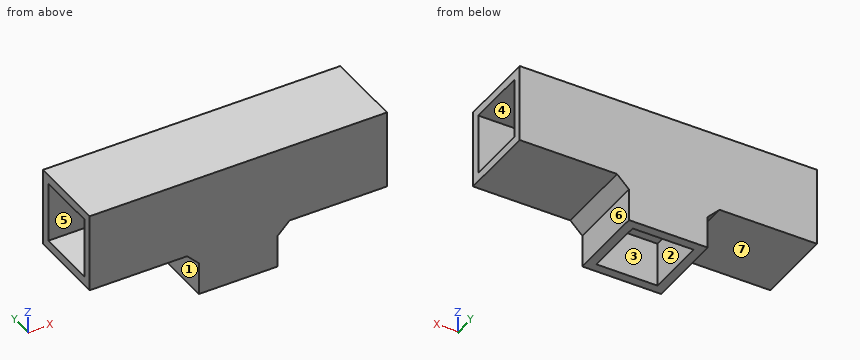
```python
from build123d import *

# Parameters (mm, degrees)
SKETCH_W      = 26.5
SKETCH_H      = 26.5
SKETCH_W_2    = 20.5
SKETCH_H_2    = 20.5
PAD_DEPTH     = 15
SKETCH001_W   = 26.5
SKETCH001_H   = 26.5
SKETCH001_W_2 = 20.5
SKETCH001_H_2 = 20.5
PAD001_DEPTH  = 50
CHAMFER_SIZE  = 4


with BuildPart() as part:
    # Sketch → Pad (new body)
    with BuildSketch(Plane.XY):
        Rectangle(SKETCH_W, SKETCH_H)
        Rectangle(SKETCH_W_2, SKETCH_H_2, mode=Mode.SUBTRACT)
    extrude(amount=PAD_DEPTH)

    # Sketch001 → Pad001 (join, symmetric)
    with BuildSketch(Plane.YZ):
        with Locations((0, 28.25)):
            Rectangle(SKETCH001_W, SKETCH001_H)
        with Locations((0, 28.25)):
            Rectangle(SKETCH001_W_2, SKETCH001_H_2, mode=Mode.SUBTRACT)
    extrude(amount=PAD001_DEPTH, both=True)

    # Chamfer
    chamfer_edges = [part.edges().sort_by_distance(p)[0] for p in [
        (13.25, 0, 15),
        (-13.25, 0, 15),
    ]]
    chamfer(chamfer_edges, length=CHAMFER_SIZE)


solid = part.part
```
The model under review builds one solid part; all positions refer to its coordinate system, in mm. Face numbers are marked on the shaded views. A direction names the side the tool comes from. Give positions to 0.01 mm unless a question says otherwise; leave off trailing zeros. Write each loop counter-clockwise with the first axis right and the second up, starting at its lowest first coordinate (ties: lowest second). Pieces come first, ordered by that corner, then holes. Notation, with made-up numbers: (-35, 43) -> (3, 43) arc R16 ccw to (3, 63) -> close; hole circle Ø7 at (43.25, -12). An arc over 180 degrees is marked (long way). Put each result on its own line as item: value.
(1) We need section D-D, the plane x = -42. Give the boundary of the cut face in (y, z), and give its area (3 significant figures).
Results are:
outline: (-13.25, 15) -> (13.25, 15) -> (13.25, 41.5) -> (-13.25, 41.5) -> close; hole (-10.25, 18) -> (10.25, 18) -> (10.25, 38.5) -> (-10.25, 38.5) -> close
area: 282 mm²
(2) For pin 1 Ø10 at (x, y) = (-1.5, -0.5) entering from -Z; pin 2 Ø9 at (y, z) = (1, 4) entering from -X; pin 3 Ø5.5 at (y, z) = (0.5, 4) entering from +X, all flat-tipped, find the tip position at first contact; note any pin that passes through.
Results are:
pin 1: z = 15
pin 2: x = -13.25
pin 3: x = 13.25
(3) We need section C-C, the plane z = 20.5. Give the boundary of the cut face in (x, y), and give its area (3 significant figures).
Results are:
outline: (-50, -13.25) -> (50, -13.25) -> (50, -10.25) -> (-50, -10.25) -> close; (-50, 10.25) -> (50, 10.25) -> (50, 13.25) -> (-50, 13.25) -> close
area: 600 mm²
(4) The part is to be moulded in two halves that separate along X. For the marked faces 1, 2, 3 and 4, say which applies: pulls with the +X half, pulls with the -X half, needs draft (parallel to the pull), parting line crosses it, or undercut.
Results are:
face 1: pulls with the -X half
face 2: undercut
face 3: undercut
face 4: needs draft
(5) Tool access review of the marked faces 5, 6 and 7: name each direction out of +Z, -Z, +X, -X, +Y, -Y from which nothing blocks a thin tool from reaching the whole face with its end or side.
Results are:
face 5: +X, -X
face 6: -Z, +X, +Y, -Y
face 7: -Z, -X, +Y, -Y
(6) We need section B-B, the plane z = 7. Give the boundary of the cut face in (x, y).
Results are:
outline: (-13.25, -13.25) -> (13.25, -13.25) -> (13.25, 13.25) -> (-13.25, 13.25) -> close; hole (-10.25, -10.25) -> (10.25, -10.25) -> (10.25, 10.25) -> (-10.25, 10.25) -> close
(7) To check wall thickness, follow probe 1 along Y at (x, z) = (36, 30); probe 2 along Z at (x, y) = (-11, -6). State the ranges of each line that lie inside material, in increasing order. Write a range as from..to.
Results are:
probe 1: -13.25..-10.25, 10.25..13.25
probe 2: 0..18, 38.5..41.5
(8) We need section A-A, the plane y = 0. Give the boundary of the cut face in (x, z).
Results are:
outline: (-50, 15) -> (-17.25, 15) -> (-13.25, 11) -> (-13.25, 0) -> (-10.25, 0) -> (-10.25, 15) -> (10.25, 15) -> (10.25, 0) -> (13.25, 0) -> (13.25, 11) -> (17.25, 15) -> (50, 15) -> (50, 18) -> (-50, 18) -> close; (-50, 38.5) -> (50, 38.5) -> (50, 41.5) -> (-50, 41.5) -> close
